Source: three-view drawing plus pictorial views. Frame: mm from the lowest corner of the part. A direction names the side the tool comes from. Coordinates: 2 decimals unless noted, no trailing zeros. Order: outer loops, then holes, each group sorted by start corner. A loop starts at its lowest first (then second) coordinate and runs counter-clockwise, first axis right, second up. Notation, with made-up numbers: (28, -7.75) -> (62, -7.75) arc R36 ccw to (62, 31.25) -> close; hole circle Ø1 at (7.25, -6). An arc over 180 degrees is marked (long way). Use one line per item in the form item = value. Start each with the question number.
1) Pin query (flat end, axial travel): pin 1 (6 mm diameter, centred on x = 6, z = 30.5, fed in from +Y); pin 2 (1.2 mm diameter, centred on y = 6, z = 28.5, fed in from -X); pin 3 (2 mm diameter, centred on y = 5, z = 25.5, fed in from +X). Return the tip coordinate at first contact, or that it passes through.
2) Section query B-B on z = 20. Output: boundary loops of the cut face in (x, y), then the cut area to 3 significant figures.
3) Section query A-A on x = 30. Output: boundary loops of the cut face in (y, z), then the cut area to 3 significant figures.
4) Section query D-D on z = 5. Output: boundary loops of the cut face in (x, y).
5) Ray query, line 1 along Z through (x, y) = (30, 2); line 2 along Y through (x, z) = (42.5, 31); line 3 along X through (y, z) = (5.5, 22.5). Return the intervals inside material, ascending.
6) Access query for the marked faces 1, 2 and 3. Directions: +Z, -Z, +X, -X, +Y, -Y. A direction counts if a zero-diameter tool reaches every point of the face in a straight line with its end or side. Return the directions, or none.
7) Section query C-C on y = 1.75. Output: boundary loops of the cut face in (x, z), then the cut area to 3 significant figures.
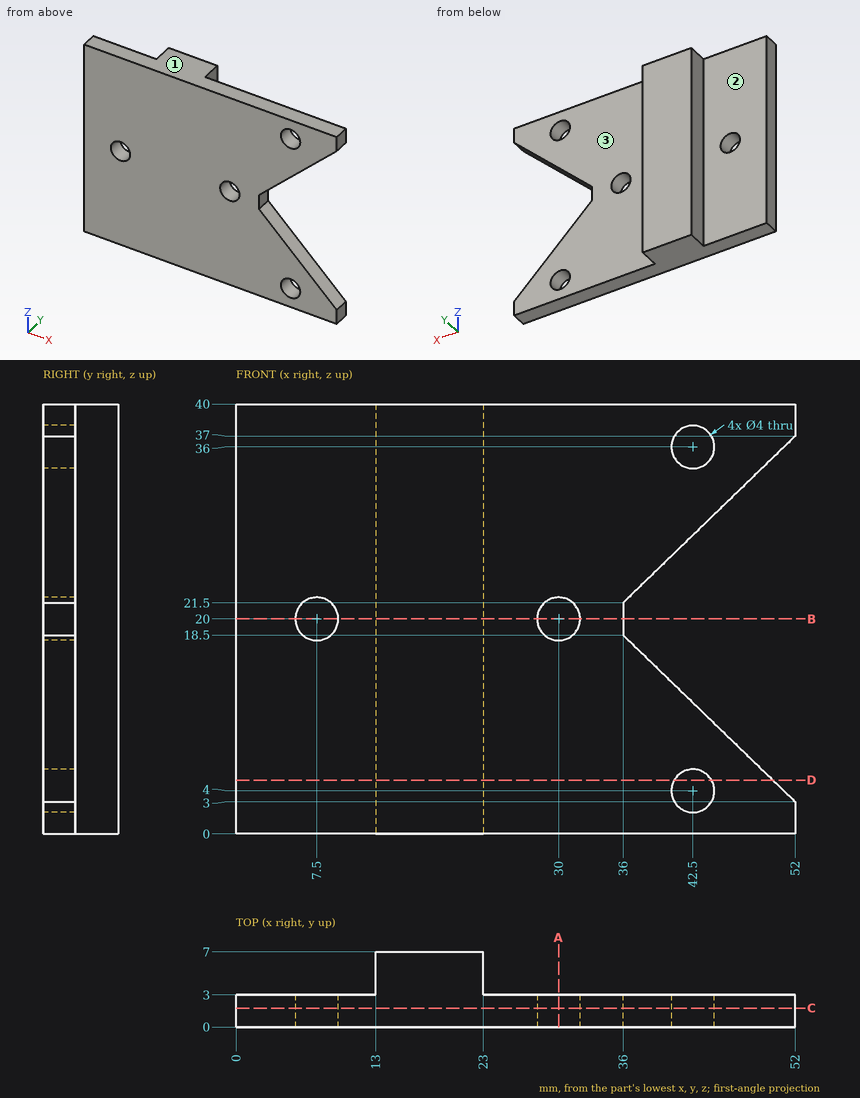
Answers below:
q1.pin_1 = 3
q1.pin_2 = 13
q1.pin_3 = 23
q2.outline = (0, 0) -> (5.5, 0) -> (5.5, 3) -> (0, 3) -> close; (9.5, 0) -> (28, 0) -> (28, 3) -> (23, 3) -> (23, 7) -> (13, 7) -> (13, 3) -> (9.5, 3) -> close; (32, 0) -> (36, 0) -> (36, 3) -> (32, 3) -> close
q2.area = 124 mm^2
q3.outline = (0, 0) -> (3, 0) -> (3, 18) -> (0, 18) -> close; (0, 22) -> (3, 22) -> (3, 40) -> (0, 40) -> close
q3.area = 108 mm^2
q4.outline = (0, 0) -> (40.77, 0) -> (40.77, 3) -> (23, 3) -> (23, 7) -> (13, 7) -> (13, 3) -> (0, 3) -> close; (44.23, 0) -> (49.94, 0) -> (49.94, 3) -> (44.23, 3) -> close
q5.line_1 = 0 to 18, 22 to 40
q5.line_2 = 0 to 3
q5.line_3 = 13 to 23
q6.face_1 = +Z, +X, -X, +Y, -Y
q6.face_2 = +Z, -Z, -X, +Y
q6.face_3 = +Z, -Z, +X, +Y
q7.outline = (0, 0) -> (52, 0) -> (52, 3) -> (36, 18.5) -> (36, 21.5) -> (52, 37) -> (52, 40) -> (0, 40) -> close; hole circle Ø4 at (7.5, 20); hole circle Ø4 at (30, 20); hole circle Ø4 at (42.5, 4); hole circle Ø4 at (42.5, 36)
q7.area = 1,730 mm^2
